Build history of the part. All positions in model axes, mm. Coordinates: 2 decimals unless noted, no trailing zeros. Order: outer loops, then holes, each group sorted by start corner. A loop starts at its lowest first (then second) coordinate and runs counter-clockwise, first axis right, second up. Notation, with made-up numbers: M 46,49 L 92,49 A16 ccw 92,73 Z; hole C 63.25,15.5 d4. An arc over 180 degrees is marked long. Write item = value, one per line. Start each with the question number.
Q1. Band-saw the part on C-C on z = -98. Write the cut outline in (x, y), plus the area to 3 significant figures.
Q2. Pin check, flat tips, straight feed: P1, Ø0.9, axis at y = -75, z = -114, coming from the +X side; P2, Ø1.5, axis at x = 53.5, y = -75, coming from the +Z side; P3, Ø1.5, axis at x = 78, y = -75, coming from the -Z side. Stop position of each tip, or through.
Q3. Band-saw the part on A-A on y = -76.05. Write the cut outline in (x, z), plus the area to 3 significant figures.
Q4. Drill centre lines: probe 1 along Z at (x, y) = (32, -74.8); probe 2 along X at (y, z) = (-75.7, -72); probe 3 along X at (y, z) = (-74.3, -106). Where is each one in solid material? Low to high.
Q5. Band-saw the part on B-B on x = 43. Write the cut outline in (y, z), plus the area to 3 significant figures.
```python
from build123d import *

# Parameters (mm, degrees)
RECTANGLE134_W                               = 40
RECTANGLE134_H                               = 3
EXTRUDE175_DEPTH                             = 3
RECTANGLE135_W                               = 40
RECTANGLE135_H                               = 3
EXTRUDE176_DEPTH                             = 3
RECTANGLE133_W                               = 40
RECTANGLE133_H                               = 3
EXTRUDE174_DEPTH                             = 3
RECTANGLE130_AS_DRAWN_W                      = 25
RECTANGLE130_AS_DRAWN_H                      = 3
EXTRUDE152_DEPTH                             = 3
EXTRUDE152_ONTO_RECTANGLE130_ROLL_ANGLE      = -90
EXTRUDE152_ONTO_RECTANGLE130_PLACEMENT_ANGLE = 180
RECTANGLE128_AS_DRAWN_W                      = 25
RECTANGLE128_AS_DRAWN_H                      = 3
EXTRUDE153_DEPTH                             = 3
EXTRUDE153_ONTO_RECTANGLE128_ROLL_ANGLE      = -90
EXTRUDE153_ONTO_RECTANGLE128_PLACEMENT_ANGLE = 180
RECTANGLE132_AS_DRAWN_W                      = 3
RECTANGLE132_AS_DRAWN_H                      = 19.5
EXTRUDE166_DEPTH                             = 3
EXTRUDE166_ONTO_RECTANGLE132_ROLL_ANGLE      = -90
EXTRUDE166_ONTO_RECTANGLE132_PLACEMENT_ANGLE = 180
RECTANGLE127_AS_DRAWN_W                      = 25
RECTANGLE127_AS_DRAWN_H                      = 3
EXTRUDE147_DEPTH                             = 3
EXTRUDE147_ONTO_RECTANGLE127_ROLL_ANGLE      = -90
EXTRUDE147_ONTO_RECTANGLE127_PLACEMENT_ANGLE = 180
RECTANGLE129_AS_DRAWN_W                      = 25
RECTANGLE129_AS_DRAWN_H                      = 3
EXTRUDE149_DEPTH                             = 3
EXTRUDE149_ONTO_RECTANGLE129_ROLL_ANGLE      = -90
EXTRUDE149_ONTO_RECTANGLE129_PLACEMENT_ANGLE = 180
BOX042_W                                     = 100
BOX042_H                                     = 3
BOX042_DEPTH                                 = 45


with BuildPart() as extrude175:
    # Rectangle134 → Extrude175 (new body)
    with BuildSketch(Plane(origin=(114, 38, -112), x_dir=(0, 1, 0), z_dir=(1, 0, 0))):
        with Locations((20, -1.5)):
            Rectangle(RECTANGLE134_W, RECTANGLE134_H)
    extrude(amount=EXTRUDE175_DEPTH)


with BuildPart() as extrude176:
    # Rectangle135 → Extrude176 (new body)
    with BuildSketch(Plane(origin=(114, -19.5, -112), x_dir=(0, 1, 0), z_dir=(1, 0, 0))):
        with Locations((20, -1.5)):
            Rectangle(RECTANGLE135_W, RECTANGLE135_H)
    extrude(amount=EXTRUDE176_DEPTH)


with BuildPart() as fusion064043:
    # Rectangle133 → Extrude174 (new body)
    with BuildSketch(Plane(origin=(114, -77, -112), x_dir=(0, 1, 0), z_dir=(1, 0, 0))):
        with Locations((20, -1.5)):
            Rectangle(RECTANGLE133_W, RECTANGLE133_H)
    extrude(amount=EXTRUDE174_DEPTH)

    # Fusion064043: union Extrude175, Extrude176
    add(extrude175.part)
    add(extrude176.part)


with BuildPart() as fusion064043_1:
    # Fusion064043 placement: moved
    add(fusion064043.part.moved(Location((-3, 0, 0))))


with BuildPart() as extrude152:
    # Rectangle130 as drawn → Extrude152 (new)
    with BuildSketch(Plane.XY):
        with Locations((12.5, 1.5)):
            Rectangle(RECTANGLE130_AS_DRAWN_W, RECTANGLE130_AS_DRAWN_H)
    extrude(amount=-EXTRUDE152_DEPTH)


with BuildPart() as extrude152_1:
    # Extrude152 onto Rectangle130 roll: moved
    add(extrude152.part.rotate(Axis((0, 0, 0), (1, 0, 0)), EXTRUDE152_ONTO_RECTANGLE130_ROLL_ANGLE))


with BuildPart() as extrude152_2:
    # Extrude152 onto Rectangle130 placement: moved
    add(extrude152_1.part.moved(Location((39, -77, -70))).rotate(Axis((39, -77, -70), (0, 0, 1)), EXTRUDE152_ONTO_RECTANGLE130_PLACEMENT_ANGLE))


with BuildPart() as extrude152_3:
    # Extrude152 placement: moved
    add(extrude152_2.part.moved(Location((0, 0, -42))))


with BuildPart() as extrude153:
    # Rectangle128 as drawn → Extrude153 (new)
    with BuildSketch(Plane.XY):
        with Locations((12.5, 1.5)):
            Rectangle(RECTANGLE128_AS_DRAWN_W, RECTANGLE128_AS_DRAWN_H)
    extrude(amount=-EXTRUDE153_DEPTH)


with BuildPart() as extrude153_1:
    # Extrude153 onto Rectangle128 roll: moved
    add(extrude153.part.rotate(Axis((0, 0, 0), (1, 0, 0)), EXTRUDE153_ONTO_RECTANGLE128_ROLL_ANGLE))


with BuildPart() as extrude153_2:
    # Extrude153 onto Rectangle128 placement: moved
    add(extrude153_1.part.moved(Location((89, -77, -70))).rotate(Axis((89, -77, -70), (0, 0, 1)), EXTRUDE153_ONTO_RECTANGLE128_PLACEMENT_ANGLE))


with BuildPart() as extrude153_3:
    # Extrude153 placement: moved
    add(extrude153_2.part.moved(Location((0, 0, -42))))


with BuildPart() as extrude166:
    # Rectangle132 as drawn → Extrude166 (new)
    with BuildSketch(Plane.XY):
        with Locations((1.5, 9.75)):
            Rectangle(RECTANGLE132_AS_DRAWN_W, RECTANGLE132_AS_DRAWN_H)
    extrude(amount=-EXTRUDE166_DEPTH)


with BuildPart() as extrude166_1:
    # Extrude166 onto Rectangle132 roll: moved
    add(extrude166.part.rotate(Axis((0, 0, 0), (1, 0, 0)), EXTRUDE166_ONTO_RECTANGLE132_ROLL_ANGLE))


with BuildPart() as extrude166_2:
    # Extrude166 onto Rectangle132 placement: moved
    add(extrude166_1.part.moved(Location((114, -77, -92.5))).rotate(Axis((114, -77, -92.5), (0, 0, 1)), EXTRUDE166_ONTO_RECTANGLE132_PLACEMENT_ANGLE))


with BuildPart() as extrude147:
    # Rectangle127 as drawn → Extrude147 (new)
    with BuildSketch(Plane.XY):
        with Locations((12.5, 1.5)):
            Rectangle(RECTANGLE127_AS_DRAWN_W, RECTANGLE127_AS_DRAWN_H)
    extrude(amount=-EXTRUDE147_DEPTH)


with BuildPart() as extrude147_1:
    # Extrude147 onto Rectangle127 roll: moved
    add(extrude147.part.rotate(Axis((0, 0, 0), (1, 0, 0)), EXTRUDE147_ONTO_RECTANGLE127_ROLL_ANGLE))


with BuildPart() as extrude147_2:
    # Extrude147 onto Rectangle127 placement: moved
    add(extrude147_1.part.moved(Location((114, -77, -70))).rotate(Axis((114, -77, -70), (0, 0, 1)), EXTRUDE147_ONTO_RECTANGLE127_PLACEMENT_ANGLE))


with BuildPart() as fusion064024:
    # Rectangle129 as drawn → Extrude149 (new)
    with BuildSketch(Plane.XY):
        with Locations((12.5, 1.5)):
            Rectangle(RECTANGLE129_AS_DRAWN_W, RECTANGLE129_AS_DRAWN_H)
    extrude(amount=-EXTRUDE149_DEPTH)


with BuildPart() as fusion064024_1:
    # Extrude149 onto Rectangle129 roll: moved
    add(fusion064024.part.rotate(Axis((0, 0, 0), (1, 0, 0)), EXTRUDE149_ONTO_RECTANGLE129_ROLL_ANGLE))


with BuildPart() as fusion064024_2:
    # Extrude149 onto Rectangle129 placement: moved
    add(fusion064024_1.part.moved(Location((64, -77, -70))).rotate(Axis((64, -77, -70), (0, 0, 1)), EXTRUDE149_ONTO_RECTANGLE129_PLACEMENT_ANGLE))

    # Fusion064024: union Extrude152, Extrude153, Extrude166, Extrude147
    add(extrude152_3.part)
    add(extrude153_3.part)
    add(extrude166_2.part)
    add(extrude147_2.part)


with BuildPart() as cut035028:
    # Box042 → Box042 (new body)
    with BuildSketch(Plane(origin=(14, -77, -115), x_dir=(1, 0, 0), z_dir=(0, 0, 1))):
        with Locations((50, 1.5)):
            Rectangle(BOX042_W, BOX042_H)
    extrude(amount=BOX042_DEPTH)

    # Cut035013: cut Fusion064024
    add(fusion064024_2.part, mode=Mode.SUBTRACT)

    # Cut035028: cut Fusion064043
    add(fusion064043_1.part, mode=Mode.SUBTRACT)


solid = cut035028.part
```
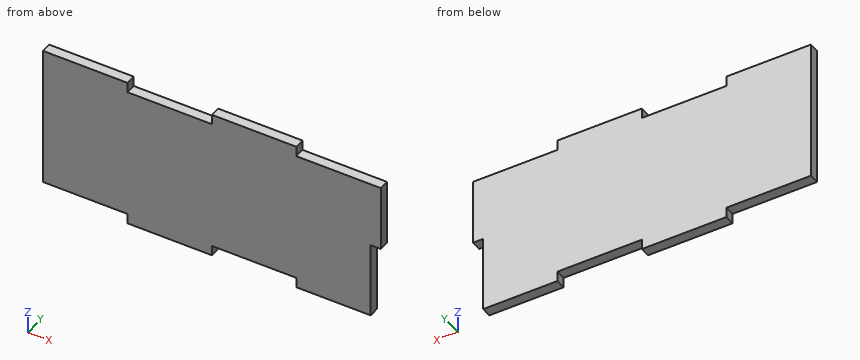
Recorded:
q1.outline = M 14,-77 L 111,-77 L 111,-74 L 14,-74 Z
q1.area = 291 mm2
q2.P1 = 111
q2.P2 = -73
q2.P3 = -112
q3.outline = M 14,-112 L 39,-112 L 39,-115 L 64,-115 L 64,-112 L 89,-112 L 89,-115 L 111,-115 L 111,-92.5 L 114,-92.5 L 114,-73 L 89,-73 L 89,-70 L 64,-70 L 64,-73 L 39,-73 L 39,-70 L 14,-70 Z
q3.area = 4,130 mm2
q4.probe_1 = -112 to -70
q4.probe_2 = 14 to 39, 64 to 89
q4.probe_3 = 14 to 111
q5.outline = M -77,-115 L -74,-115 L -74,-73 L -77,-73 Z
q5.area = 126 mm2
